The drawing under review shows one solid part. Ordinate dimensions are in mm from its lowest x, y, z. A direction names the side the tool comes from. Round coordinates to 2 decimals unless told otherwise and drop trailing zeros. Loops run counter-clockwise (first coordinate to the right, second up) from the corner with the lowest first, then second, coordinate; pieces in that order, holes last. Notation, with made-up numbers: M 29,40.5 L 61,40.5 A12 cw 61,58.5 Z; hole C -1,17.5 d11. An arc over 180 degrees is marked long. Use a Markdown table: item, result.
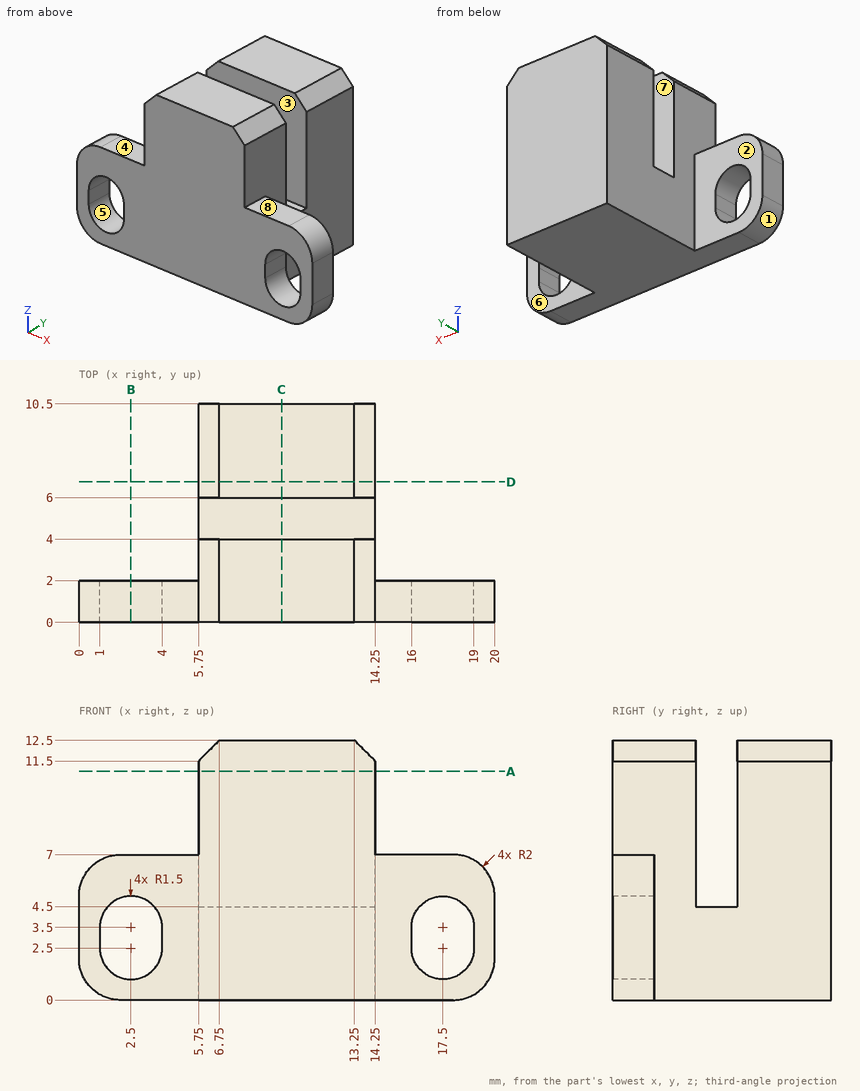
1. Take a section at A-A on z = 11. Give the boundary of the cut face in (x, y), and give its area (4 significant figures).
Check values:
| item | result |
|---|---|
| outline | M 5.75,0 L 14.25,0 L 14.25,4 L 5.75,4 Z; M 5.75,6 L 14.25,6 L 14.25,10.5 L 5.75,10.5 Z |
| area | 72.25 mm² |
2. Wall thickness on line 1 along X through (y, z) = (1, 3); line 2 along Y through (x, z) = (12.5, 12.25); line 3 along X through (y, z) = (1, 4): over which ranges is each line inside the solid? List them lowest first. Write a range as from..to.
Check values:
| item | result |
|---|---|
| line 1 | x = 0..1, 4..16, 19..20 |
| line 2 | y = 0..4, 6..10.5 |
| line 3 | x = 0..1.09, 3.91..16.09, 18.91..20 |
3. Take a section at B-B on x = 2.5. Give the boundary of the cut face in (y, z).
Check values:
| item | result |
|---|---|
| outline | M 0,0 L 2,0 L 2,1 L 0,1 Z; M 0,5 L 2,5 L 2,7 L 0,7 Z |
4. Take a section at C-C on x = 9.75. Give the boundary of the cut face in (y, z), and give its area (3 significant figures).
Check values:
| item | result |
|---|---|
| outline | M 0,0 L 10.5,0 L 10.5,12.5 L 6,12.5 L 6,4.5 L 4,4.5 L 4,12.5 L 0,12.5 Z |
| area | 115 mm² |
5. Machinability: for the marked faces 4, 5, 6, 7 and 8, which of the approach directions +Z, -Z, +X, -X, +Y, -Y give a long, thin tool a straight path to every point of the face, cutting with its end or side? Answer none if there is none.
Check values:
| item | result |
|---|---|
| face 4 | +Z, -X, +Y, -Y |
| face 5 | +Y, -Y |
| face 6 | +Z, -Z, +X, +Y |
| face 7 | +Z, +X, -X |
| face 8 | +Z, +X, +Y, -Y |
6. Insertion check: pin 1 (2 mm diameter, centred on x = 16, z = 5, fed in from +Y); pin 2 (1 mm diameter, centred on x = 9.5, y = 5, fed in from +Z); pin 3 (0.6 mm diameter, centred on x = 15.5, y = 1.5, fed in from +Z). Each pin has a flat end and moves straight along its axis. Give the tip position at first contact, or say it passes through.
Check values:
| item | result |
|---|---|
| pin 1 | stops at y = 2 |
| pin 2 | stops at z = 4.5 |
| pin 3 | stops at z = 7 |
7. Take a section at D-D on y = 6.75. Give the boundary of the cut face in (x, z), and give its area (3 significant figures).
Check values:
| item | result |
|---|---|
| outline | M 5.75,0 L 14.25,0 L 14.25,11.5 L 13.25,12.5 L 6.75,12.5 L 5.75,11.5 Z |
| area | 105 mm² |
8. The part is to be moulded in two halves that separate along Y. For the marked faces 1, 2 and 3, say which applies: pulls with the +Y half, pulls with the -Y half, needs draft (parallel to the pull), parting line crosses it, or undercut.
Check values:
| item | result |
|---|---|
| face 1 | needs draft |
| face 2 | pulls with the +Y half |
| face 3 | undercut |
